```python
from build123d import *

# Parameters (mm, degrees)
BOSS_EXTRUDE1_DEPTH = 10
SKETCH2_R           = 1.75
CUT_EXTRUDE1_DEPTH  = 10
SKETCH3_R           = 1.25
SKETCH3_R_2         = 1.8
CUT_EXTRUDE2_DEPTH  = 40.143965052
SKETCH4_W           = 13.022509218
SKETCH4_H           = 4.5
CUT_EXTRUDE3_DEPTH  = 40.143965052


with BuildPart() as part:
    # Sketch1 → Boss-Extrude1 (new body)
    with BuildSketch(Plane.XY):
        Polygon((0, 0), (0, 36.5), (12.5, 36.5), (12.5, 34), (2.5, 34), (2.5, 0), align=None)
    extrude(amount=BOSS_EXTRUDE1_DEPTH)

    # Sketch2 → Cut-Extrude1 (cut)
    with BuildSketch(Plane.XZ.offset(-34)):
        with Locations((7.5, 5)):
            Circle(SKETCH2_R)
    extrude(amount=-CUT_EXTRUDE1_DEPTH, mode=Mode.SUBTRACT)

    # Sketch3 → Cut-Extrude2 (cut, through all)
    with BuildSketch(Plane(origin=(2.5, 0, 0), x_dir=(0, 0, -1), z_dir=(1, 0, 0))):
        with Locations(Location((-3.25, 7.15, 0), (0, 0, 90))):
            Circle(SKETCH3_R)
        with Locations(Location((-3.25, 16.85, 0), (0, 0, 270))):
            Circle(SKETCH3_R)
        with Locations(Location((-5, 29, 0), (0, 0, 90))):
            Circle(SKETCH3_R_2)
    extrude(amount=-CUT_EXTRUDE2_DEPTH, mode=Mode.SUBTRACT)

    # Sketch4 → Cut-Extrude3 (cut, through all)
    with BuildSketch(Plane(origin=(2.5, 0, 0), x_dir=(0, 0, -1), z_dir=(1, 0, 0))):
        with Locations((-6.511254609, 2.25)):
            Rectangle(SKETCH4_W, SKETCH4_H)
    extrude(amount=-CUT_EXTRUDE3_DEPTH, mode=Mode.SUBTRACT)


solid = part.part
```
Geometry check sheet. Reference: the model listing, model coordinates, mm. A direction names the side the tool comes from. Coordinates: 2 decimals unless noted, no trailing zeros. Order: outer loops, then holes, each group sorted by start corner. A loop starts at its lowest first (then second) coordinate and runs counter-clockwise, first axis right, second up. Notation, with made-up numbers: (80.5, 74.5) - (132.5, 74.5) arc R30 ccw to (132.5, 103.5) - close; hole circle Ø6 at (-29.75, -22.75). An arc over 180 degrees is marked (long way). Answer in a Markdown table with one row per item. Add a question column.
1. Section check D-D (x = 8.25). Enter the section's corners in (y, z), plus the area to 3 significant figures.
2. Draft check along Z on faces 3 (the face through (1.268, 15.695, 3.729)), 4 (the face through (1.3, 5.9, 3.3)), 5 (the face through (2, 24, 10)), 6 (the face through (10, 34, 5)). Enter one of: +Z half, -Z half, draft (parallel to the pull), parting line (faces both ways), or undercut.
3. Material ranges on L1, parallel to Z at x = 7.5, y = 35.2; L2, parallel to X at y = 28, z = 2; L3, parallel to Y at x = 11, z = 4.75, recorded low to high. Write a range as [from, to].
4. Access from +Z, -Z, +X, -X, +Y, -Y to the whole of each face (thin tool, end or side, straight path). Record for faces 1 (the face through (2.5, 19, 5)), 2 (the face through (5, 36.5, 5)).
5. Section check B-B (x = 1.75). Enter the section's corners in (y, z).
6. Section check C-C (z = 5). Enter the section's corners in (x, y).
7. Section check A-A (y = 16.85). Enter the section's corners in (x, z), plus the area to 4 significant figures.
8. Gauge pin test, flat ends, axial feed: pin 1 Ø3 at (x, z) = (9, 4.5) entering from -Y; pin 2 Ø3 at (y, z) = (23, 7) entering from +X. Record the tip position at first contact, or that the pin passes through.
Data:
| question | item | result |
|---|---|---|
| 1 | outline | (34, 0) - (36.5, 0) - (36.5, 3.42) - (34, 3.42) - close; (34, 6.58) - (36.5, 6.58) - (36.5, 10) - (34, 10) - close |
| 1 | area | 17.1 mm² |
| 2 | face 3 | undercut |
| 2 | face 4 | undercut |
| 2 | face 5 | +Z half |
| 2 | face 6 | draft |
| 3 | L1 | z = [0, 3.25], [6.75, 10] |
| 3 | L2 | x = [0, 2.5] |
| 3 | L3 | y = [34, 36.5] |
| 4 | face 1 | +Z, -Z, +X, -Y |
| 4 | face 2 | +Z, -Z, +X, -X, +Y |
| 5 | outline | (4.5, 0) - (36.5, 0) - (36.5, 10) - (4.5, 10) - close; hole circle Ø2.5 at (7.15, 3.25); hole circle Ø2.5 at (16.85, 3.25); hole circle Ø3.6 at (29, 5) |
| 6 | outline | (0, 4.5) - (2.5, 4.5) - (2.5, 27.2) - (0, 27.2) - close; (0, 30.8) - (2.5, 30.8) - (2.5, 34) - (5.75, 34) - (5.75, 36.5) - (0, 36.5) - close; (9.25, 34) - (12.5, 34) - (12.5, 36.5) - (9.25, 36.5) - close |
| 7 | outline | (0, 0) - (2.5, 0) - (2.5, 2) - (0, 2) - close; (0, 4.5) - (2.5, 4.5) - (2.5, 10) - (0, 10) - close |
| 7 | area | 18.75 mm² |
| 8 | pin 1 | stops at y = 34 |
| 8 | pin 2 | stops at x = 2.5 |
